from build123d import *

# Parameters (mm, degrees)
SKETCH1_W          = 11
SKETCH1_H          = 7.62
SKETCH2_R          = 2.54
CUT_EXTRUDE1_DEPTH = 33.032240009
SKETCH3_R          = 3.96875
CUT_EXTRUDE2_DEPTH = 5.08


with BuildPart() as part:
    # Sketch1 → Revolve1 (revolve)
    with BuildSketch(Plane.XY, mode=Mode.PRIVATE) as revolve1_sk:
        with Locations((16.5, -29.147212191)):
            Rectangle(SKETCH1_W, SKETCH1_H)
    revolve(revolve1_sk.sketch.rotate(Axis((0, 18.662787809, 0), (0, -1, 0)), 180), axis=Axis((0, 18.662787809, 0), (0, -1, 0)))

    # Sketch2 → Cut-Extrude1 (cut, through all)
    with BuildSketch(Plane.XZ.offset(32.957212191)):
        with Locations((15.074245783, 4.897919361)):
            Circle(SKETCH2_R)
        with Locations((0, 15.85)):
            Circle(SKETCH2_R)
        with Locations((9.316396249, -12.822919361)):
            Circle(SKETCH2_R)
        with Locations((-9.316396249, -12.822919361)):
            Circle(SKETCH2_R)
        with Locations((-15.074245783, 4.897919361)):
            Circle(SKETCH2_R)
    extrude(amount=-CUT_EXTRUDE1_DEPTH, mode=Mode.SUBTRACT)

    # Sketch3 → Cut-Extrude2 (cut)
    with BuildSketch(Plane(origin=(0, -32.957212191, 0), x_dir=(-1, 0, 0), z_dir=(0, -1, 0))):
        with Locations(Location((0, -15.85, 0), (0, 0, 180))):
            Circle(SKETCH3_R)
        with Locations(Location((-15.074245783, -4.897919361, 0), (0, 0, 180))):
            Circle(SKETCH3_R)
        with Locations(Location((-9.316396249, 12.822919361, 0), (0, 0, 180))):
            Circle(SKETCH3_R)
        with Locations(Location((9.316396249, 12.822919361, 0), (0, 0, 180))):
            Circle(SKETCH3_R)
        with Locations(Location((15.074245783, -4.897919361, 0), (0, 0, 180))):
            Circle(SKETCH3_R)
    extrude(amount=-CUT_EXTRUDE2_DEPTH, mode=Mode.SUBTRACT)


solid = part.part
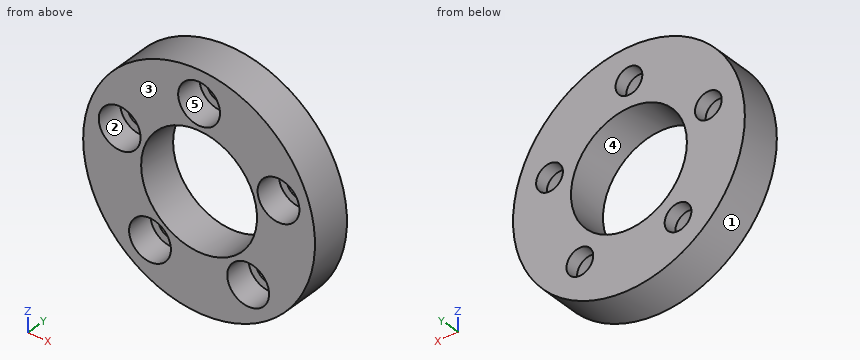
Read the model definition and answer for the solid it produces. Units are mm, in the model's axes. Face numbers are marked on the shaded views. A direction names the side the tool comes from. Give positions to 0.01 mm unless a question says otherwise; leave off trailing zeros. Loops run counter-clockwise (first coordinate to the right, second up) from the corner with the lowest first, then second, coordinate; pieces in that order, holes last. Notation, with made-up numbers: (6, 60.25) -> (39, 60.25) arc R31 ccw to (39, 85.25) -> close; hole circle Ø5 at (-21, 9). An arc over 180 degrees is marked (long way). Use a Markdown table: item, result.
Q1. Section A-A, the plane x = 0 is taken. Determine the outline of the cut face in (y, z), then the cut area to 3 significant figures.
Solved:
| item | result |
|---|---|
| outline | (-32.96, -22) -> (-25.34, -22) -> (-25.34, -11) -> (-32.96, -11) -> close; (-32.96, 11) -> (-25.34, 11) -> (-25.34, 13.31) -> (-27.88, 13.31) -> (-27.88, 11.88) -> (-32.96, 11.88) -> close; (-32.96, 19.82) -> (-27.88, 19.82) -> (-27.88, 18.39) -> (-25.34, 18.39) -> (-25.34, 22) -> (-32.96, 22) -> close |
| area | 114 mm^2 |
Q2. Determine the mould class of the marked faces 1, 2 and 3 for opening direction Z: pulls with the +Z half, pulls with the -Z half, needs draft (parallel to the pull), parting line crosses it, or undercut.
Solved:
| item | result |
|---|---|
| face 1 | parting line crosses it |
| face 2 | undercut |
| face 3 | needs draft |
Q3. Section C-C, the plane z = -12 is taken. Determine the outline of the cut face in (x, y), then the cut area to 3 significant figures.
Solved:
| item | result |
|---|---|
| outline | (-18.44, -32.96) -> (-13.2, -32.96) -> (-13.2, -27.88) -> (-11.72, -27.88) -> (-11.72, -25.34) -> (-18.44, -25.34) -> close; (-6.91, -27.88) -> (-5.43, -27.88) -> (-5.43, -32.96) -> (5.43, -32.96) -> (5.43, -27.88) -> (6.91, -27.88) -> (6.91, -25.34) -> (-6.91, -25.34) -> close; (11.72, -27.88) -> (13.2, -27.88) -> (13.2, -32.96) -> (18.44, -32.96) -> (18.44, -25.34) -> (11.72, -25.34) -> close |
| area | 178 mm^2 |
Q4. Section D-D, the plane x = -16 is taken. Determine the outline of the cut face in (y, z).
Solved:
| item | result |
|---|---|
| outline | (-32.96, -15.1) -> (-25.34, -15.1) -> (-25.34, 2.53) -> (-27.88, 2.53) -> (-27.88, 1.04) -> (-32.96, 1.04) -> close; (-32.96, 8.76) -> (-27.88, 8.76) -> (-27.88, 7.26) -> (-25.34, 7.26) -> (-25.34, 15.1) -> (-32.96, 15.1) -> close |
Q5. A tool of negligible diameter and unlimited length cuts with its end or side. For the marked faces 4 and 5, from which of +Z, -Z, +X, -X, +Y, -Y can it reach the whole face along a straight path? Write none if from no direction.
Solved:
| item | result |
|---|---|
| face 4 | +Y, -Y |
| face 5 | -Y |
Q6. Each of these flat-tipped pins is pushed along its axis until it touches: pin 1 (1.5 mm diameter, centred on x = -10.5, y = -28.5, fed in from +Z); pin 2 (3 mm diameter, centred on y = -28, z = 5.5, fed in from +X); pin 3 (1 mm diameter, centred on x = 0, y = -31.5, fed in from +Z). Where does it stop, or does it pass through?
Solved:
| item | result |
|---|---|
| pin 1 | stops at z = 19.72 |
| pin 2 | stops at x = 21.63 |
| pin 3 | stops at z = 22 |
Q7. Section B-B, the plane z = 0 is taken. Determine the outline of the cut face in (x, y).
Solved:
| item | result |
|---|---|
| outline | (-22, -32.96) -> (-11, -32.96) -> (-11, -25.34) -> (-22, -25.34) -> close; (11, -32.96) -> (22, -32.96) -> (22, -25.34) -> (11, -25.34) -> close |
Q8. Find the intervals of material crossed by line 1 along Z through (x, y) = (0, -27.2); line 2 along Z through (x, y) = (0, -32.5); line 3 along X through (y, z) = (-31.5, -14), in increasing order.
Solved:
| item | result |
|---|---|
| line 1 | z = -22 to -11, 11 to 13.31, 18.39 to 22 |
| line 2 | z = -22 to -11, 11 to 11.88, 19.82 to 22 |
| line 3 | x = -16.97 to -13.11, -5.53 to 5.53, 13.11 to 16.97 |
